from build123d import *

# Parameters (mm, degrees)
BASE_EXTRUDE_DEPTH = 3


with BuildPart() as part:
    # Sketch1 → Base-Extrude (new body)
    with BuildSketch(Plane.XY):
        with BuildLine():
            Line((570.053994223, -52.227879558), (555.477414106, -52.227879558))
            Line((555.477414106, -52.227879558), (542.114900608, -58.051960683))
            ThreePointArc((542.114900608, -58.051960683), (540.467412221, -70.727788214), (542.114985017, -83.403604775))
            Line((542.114985017, -83.403604775), (555.477414106, -89.227879558))
            Line((555.477414106, -89.227879558), (570.053994223, -89.227879558))
            Line((570.053994223, -89.227879558), (570.053994223, -86.227879558))
            Line((570.053994223, -86.227879558), (590.053994223, -86.227879558))
            Line((590.053994223, -86.227879558), (590.053994223, -70.727623116))
            Line((590.053994223, -70.727623116), (590.053994223, -55.227879558))
            Line((590.053994223, -55.227879558), (570.053994223, -55.227879558))
            Line((570.053994223, -55.227879558), (570.053994223, -52.227879558))
        make_face()
    extrude(amount=BASE_EXTRUDE_DEPTH)


solid = part.part
The model under review builds one solid part; all positions refer to its coordinate system, in mm. A direction names the side the tool comes from. Give positions to 0.01 mm unless a question says otherwise; leave off trailing zeros. Order: outer loops, then holes, each group sorted by start corner. A loop starts at its lowest first (then second) coordinate and runs counter-clockwise, first axis right, second up. Notation, with made-up numbers: M 32.25,10.5 L 43.25,10.5 A10 cw 43.25,26.5 Z; hole C 14,85.5 d4. An arc over 180 degrees is marked long. One line per question, with ' | ' between items. Start each with the question number.
1) Consider section C-C, the plane y = -82. Give the boundary of the cut face in (x, z).
2) Consider section A-A, the plane z = 0.85. Give the boundary of the cut face in (x, y), then the cut area to 3 significant figures.
3) Consider section B-B, the plane x = 575.5. Give the boundary of the cut face in (y, z).
4) For faces 1 (the face through (565, -70, 0)), 2 (the face through (580, -86.228, 1)), 3 (the face through (580, -55.228, 1)), list the 3-axis set-ups (+Z, -Z, +X, -X, +Y, -Y) from which the entire face can be reached by the end or side of a thin tool; tool diameter is ignored.
5) Clearance check with flat-ended pins moving along their axes: P1, Ø1.5, axis at y = -87.5, z = 1, coming from the +X side; P2, Ø0.9, axis at x = 584, z = 1.5, coming from the -Y side. State where each tip first meets the part, or that it passes through.
6) Wall thickness on L1, parallel to X at y = -70.5, z = 1.95; L2, parallel to Y at x = 586, z = 0.9; L3, parallel to X at y = -65.5, z = 0.9: over which ranges is each line inside the solid? List them lowest first. Write a range as from..to.
Found:
1) outline: M 541.77,0 L 590.05,0 L 590.05,3 L 541.77,3 Z
2) outline: M 542.11,-83.4 L 555.48,-89.23 L 570.05,-89.23 L 570.05,-86.23 L 590.05,-86.23 L 590.05,-55.23 L 570.05,-55.23 L 570.05,-52.23 L 555.48,-52.23 L 542.11,-58.05 A49.59 ccw Z | area: 1,600 mm²
3) outline: M -86.23,0 L -55.23,0 L -55.23,3 L -86.23,3 Z
4) face 1: -Z, +X, -X, +Y, -Y | face 2: +Z, -Z, +X, -Y | face 3: +Z, -Z, +X, +Y
5) P1: stops at x = 570.05 | P2: stops at y = -86.23
6) L1: x = 540.47..590.05 | L2: y = -86.23..-55.23 | L3: x = 540.74..590.05
